Check sheet for the modelled part. Datum: model origin and axes. Units: mm. Face numbers are marked on the shaded views. Coordinates: 2 decimals unless noted, no trailing zeros. Write each loop counter-clockwise with the first axis right and the second up, starting at its lowest first coordinate (ties: lowest second). Pieces come first, ordered by that corner, then holes. Notation, with made-up numbers: (-21.75, -12.75) -> (-10.75, -12.75) arc R21 cw to (-10.75, -7.75) -> close; hole circle Ø8 at (0, -4). An arc over 180 degrees is marked (long way). Put each result on its own line as item: value.
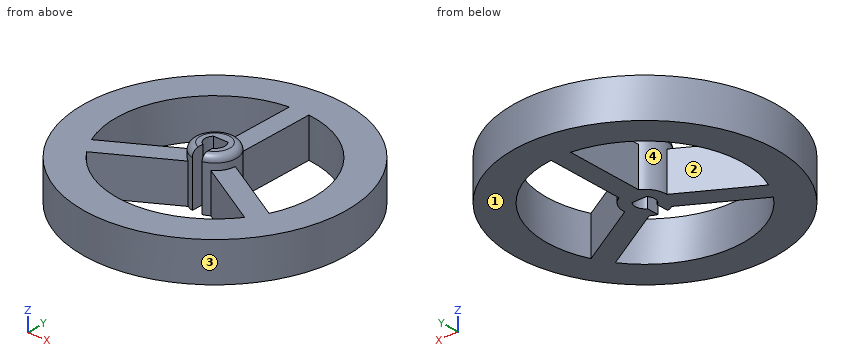
Autodesk Inventor part; units mm, degrees
ref_plane "YZ Plane" through (0, 0, 0) normal (1, 0, 0) x (0, 1, 0)
ref_plane "XZ Plane" through (0, 0, 0) normal (0, 1, 0) x (-1, 0, 0)
ref_plane "XY Plane" through (0, 0, 0) normal (0, 0, 1) x (1, 0, 0)
sketch "Эскиз1" plane through (0, 0, 0) normal (0, 0, 1) x (1, 0, 0)
  circle A0 centre (0, 0) radius 20
  circle A1 centre (0, 0) radius 15
  circle A2 centre (0, 0) radius 3.25
  line L0 (0, 15) -> (12.9904, -7.5)
  line L1 (12.9904, -7.5) -> (-12.9904, -7.5)
  line L2 (-12.9904, -7.5) -> (0, 15)
  line L3 (1.5, -15) -> (1.5, 15)
  line L4 (1.5, 15) -> (-1.5, 15)
  line L5 (-1.5, 15) -> (-1.5, -15)
  line L6 (-1.5, -15) -> (1.5, -15)
  line L7 (1.5, -15) -> (-1.5, 15) construction
  line L8 (1.5, 15) -> (-1.5, -15) construction
  line L9 (13.7404, 6.201) -> (-12.2404, -8.799)
  line L10 (-12.2404, -8.799) -> (-13.7404, -6.201)
  line L11 (-13.7404, -6.201) -> (12.2404, 8.799)
  line L12 (12.2404, 8.799) -> (13.7404, 6.201)
  line L13 (13.7404, 6.201) -> (-13.7404, -6.201) construction
  line L14 (-12.2404, -8.799) -> (12.2404, 8.799) construction
  line L15 (-13.7404, 6.201) -> (12.2404, -8.799)
  line L16 (12.2404, -8.799) -> (13.7404, -6.201)
  line L17 (13.7404, -6.201) -> (-12.2404, 8.799)
  line L18 (-12.2404, 8.799) -> (-13.7404, 6.201)
  line L19 (-13.7404, 6.201) -> (13.7404, -6.201) construction
  line L20 (12.2404, -8.799) -> (-12.2404, 8.799) construction
  point P0 (1.5, 14.9248)
  point P1 (13.6753, -6.1634)
  point P2 (3.2469, -0.1425)
  point P3 (1.5, 2.8831)
  point P4 (1.7469, -2.7406)
  point P5 (12.1753, -8.7614)
  point P6 (-12.1753, -8.7614)
  point P7 (-1.7469, -2.7406)
  point P8 (-1.5, 14.9248)
  point P9 (-1.5, 2.8831)
  point P10 (-3.2469, -0.1425)
  point P11 (-13.6753, -6.1634)
  dimension "d1" = 30
  dimension "d0" = 40
  dimension "d2" = 6.5
  dimension "d3" = 3
  dimension "d4" = 3
  dimension "d5" = 3
extrude "Выдавливание1" add sketch "Эскиз1" along normal blind 6 contours A0 | A1 L12 L9 | L17 L16 A1 | A1 L0 L17 | A1 L11 L12 | L16 L15 A1 | L1 L15 A2 L17 L0 | A1 L15 L1 | L9 L17 L3 L11 A2 | A2 L17 L9 | A2 L15 L3 L9 L17 | L3 L0 A1 | A1 L4 L3 | L3 A2 L5 L2 L0 | L11 L3 A2 | L9 L3 L17 | L3 L6 A1 | A2 L3 L15 | L2 L5 A1 | A1 L5 L4 | L3 L11 L17 L5 A2 | L3 L17 L11 | L9 L15 L5 L11 L17 L3 | L3 L15 L9 | L6 L5 A1 | A2 L5 L9 L15 L3 | L5 L17 A2 | L11 L5 L17 | L9 L5 L15 | L9 A1 L1 | L1 L2 L11 A2 L9 | A2 L9 L5 | A1 L18 L17 | L17 L5 L11 L15 A2 | L5 L15 L11 | L9 A2 L11 L15 L5 | L9 L10 A1 | L10 L11 A1 | A1 L11 L2 | A1 L15 L18 | L15 L11 A2
sketch "Эскиз2" plane through (0, 0, 6) normal (0, 0, 1) x (1, 0, 0)
  circle A0 centre (0, 0) radius 3.25
extrude "Выдавливание2" add sketch "Эскиз2" along normal blind 2
sketch "Эскиз3" plane through (0, 0, 8) normal (0, 0, 1) x (1, 0, 0)
  circle A0 centre (0, 0) radius 1.5
  line L0 (-1.5, -1) -> (1.5, -1)
  line L1 (1.5, -1) -> (1.5, 1)
  line L2 (1.5, 1) -> (-1.5, 1)
  line L3 (-1.5, 1) -> (-1.5, -1)
  line L4 (-1.5, -1) -> (1.5, 1) construction
  line L5 (1.5, -1) -> (-1.5, 1) construction
  line L6 (0.75, 3.2651) -> (-0.75, 3.2651)
  line L7 (-0.75, 3.2651) -> (-0.75, -3.2651)
  line L8 (-0.75, -3.2651) -> (0.75, -3.2651)
  line L9 (0.75, -3.2651) -> (0.75, 3.2651)
  line L10 (0.75, 3.2651) -> (-0.75, -3.2651) construction
  line L11 (-0.75, 3.2651) -> (0.75, -3.2651) construction
  point P0 (-1.118, 1)
  point P1 (-0.75, -1.299)
  point P2 (0.75, -1.299)
  point P3 (1.118, 1)
  dimension "d10" = 3
  dimension "d11" = 2
  dimension "d12" = 1.5
extrude "Выдавливание3" cut sketch "Эскиз3" against normal through all contours A0 L0 L9 L2 | A0 L9 L0 | L9 L0 L7 L2 | L9 L8 L7 A0 | A0 L7 L0 L9 | L7 L0 A0 L2 | A0 L0 L7
fillet "Сопряжение1" radius 1 1 edges at (-3.25, 0, 8)
properties part number "Колесо D40 под ось моторов серии N"
Q1. Mould release check, pull along Y, two halves, no side actions. Record for the marked faces 1, 2, 3 and 4: released by +Y, released by -Y, zero draft, split by the parting line, or undercut.
Recorded:
face 1: zero draft
face 2: undercut
face 3: split by the parting line
face 4: undercut
Q2. Cross-section at D-D (x = -8.5). Record the cut outline in (y, z).
Recorded:
outline: (-18.1, 0) -> (-12.36, 0) -> (-12.36, 6) -> (-18.1, 6) -> close; (-6.64, 0) -> (-3.18, 0) -> (-3.18, 6) -> (-6.64, 6) -> close; (12.36, 0) -> (18.1, 0) -> (18.1, 6) -> (12.36, 6) -> close
Q3. Depth check by flat-ended pin: P1, Ø2.5, axis at x = 0.5, z = 2.5, coming from the -Y side; P2, Ø2, axis at x = 13.5, y = 9, coming from the +Z side; P3, Ø0.6, axis at y = -2, z = 5.5, coming from the -X side. Enter the tip coordinate at first touch or a pass-through.
Recorded:
P1: stops at y = -20
P2: stops at z = 6
P3: stops at x = -19.93
Q4. Cross-section at C-C (z = 5.5). Record the cut outline in (x, y).
Recorded:
outline: circle Ø40 at (0, 0); hole (-13.68, -6.16) -> (-3.25, -0.14) arc R3.25 cw to (-1.5, 2.88) -> (-1.5, 14.92) arc R15 ccw to start; hole (-12.18, -8.76) arc R15 ccw to (12.18, -8.76) -> (1.75, -2.74) arc R3.25 cw to (0.75, -3.16) -> (0.75, -1.3) arc R1.5 ccw to (1.12, 1) -> (-1.12, 1) arc R1.5 ccw to (-0.75, -1.3) -> (-0.75, -3.16) arc R3.25 cw to (-1.75, -2.74) -> close; hole (1.5, 2.88) arc R3.25 cw to (3.25, -0.14) -> (13.68, -6.16) arc R15 ccw to (1.5, 14.92) -> close
Q5. Cross-section at A-A (x = 0). Record the cut outline in (y, z).
Recorded:
outline: (-20, 0) -> (-15, 0) -> (-15, 6) -> (-20, 6) -> close; (1, 0) -> (20, 0) -> (20, 6) -> (3.25, 6) -> (3.25, 7) arc R1 ccw to (2.25, 8) -> (1, 8) -> close
Q6. Material ranges on line 1 along Y through (x, z) = (-5, 1); line 2 along X through (y, z) = (-4, 2); line 3 along X through (y, z) = (3.5, 5.5), recorded low to high.
Recorded:
line 1: y = -19.36 to -14.14, -4.62 to -1.15, 14.14 to 19.36
line 2: x = -19.6 to -14.46, -9.93 to -3.93, 3.93 to 9.93, 14.46 to 19.6
line 3: x = -19.69 to -14.59, -1.5 to 1.5, 14.59 to 19.69
Q7. Cross-section at B-B (y = 12). Record the cut outline in (x, z).
Recorded:
outline: (-16, 0) -> (-9, 0) -> (-9, 6) -> (-16, 6) -> close; (-1.5, 0) -> (1.5, 0) -> (1.5, 6) -> (-1.5, 6) -> close; (9, 0) -> (16, 0) -> (16, 6) -> (9, 6) -> close
